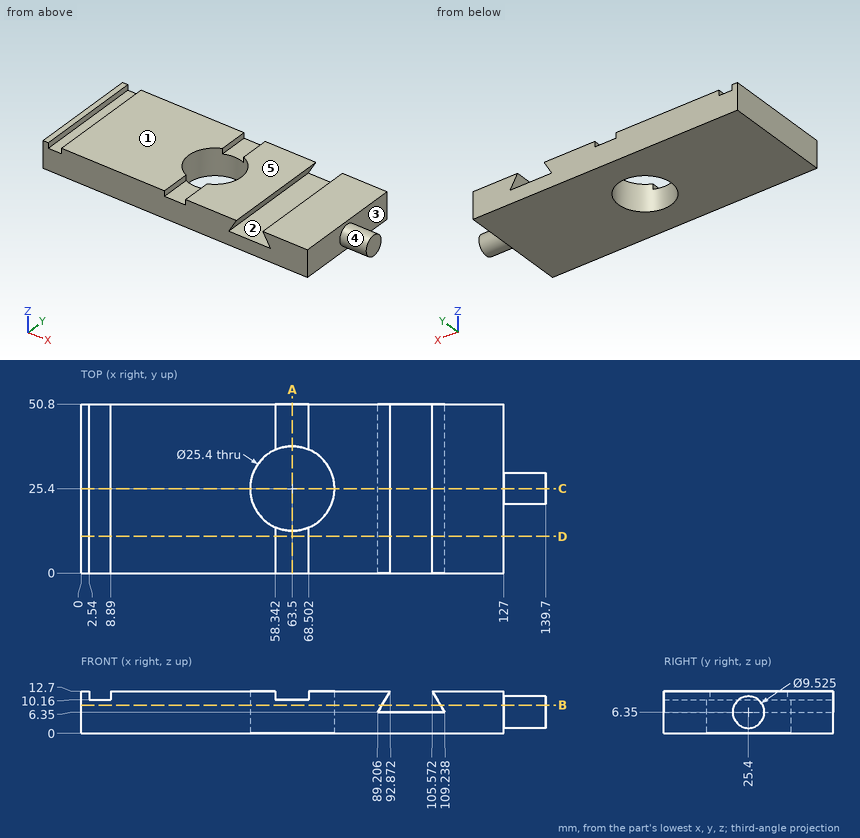
Part print with two shaded views. Sizes in mm from the minimum x, y, z corner. A direction names the side the tool comes from. Round coordinates to 2 decimals unless told otherwise and drop trailing zeros. Write each loop counter-clockwise with the first axis right and the second up, starting at its lowest first coordinate (ties: lowest second). Pieces come first, ordered by that corner, then holes. Notation, with made-up numbers: (77.5, 33) - (136.5, 33) arc R36 ccw to (136.5, 71) - close; hole circle Ø5 at (22, 18). An arc over 180 degrees is marked (long way). Answer as CSV lines item,"result".
Q1. Cut at B-B (z = 8.5). Write the cut outline in (x, y), and give its area (3 significant figures).
Report:
outline,"(0, 0) - (90.45, 0) - (90.45, 50.8) - (0, 50.8) - close; (108, 0) - (127, 0) - (127, 21.15) - (139.7, 21.15) - (139.7, 29.65) - (127, 29.65) - (127, 50.8) - (108, 50.8) - close; hole circle Ø25.4 at (63.5, 25.4)"
area,"5,160 mm^2"
Q2. Drop flat-ended pins along their axis: pin 1 (5 mm diameter, centred on x = 62.5, y = 5, fed in from +Z); pin 2 (3 mm diameter, centred on y = 30.5, z = 11.5, fed in from +X). Give the stop position or say it passes through.
Report:
pin 1,"stops at z = 10.16"
pin 2,"stops at x = 127"
Q3. Tool access for the marked faces 4 and 5: list every direction of +Z, -Z, +X, -X, +Y, -Y with a clear straight run to the whole face (end or side of a thin tool).
Report:
face 4,"+X"
face 5,"+Z, +X, -X, +Y, -Y"
Q4. Cut at A-A (x = 63.5). Write the cut outline in (y, z), and give its area (3 significant figures).
Report:
outline,"(0, 0) - (12.7, 0) - (12.7, 10.16) - (0, 10.16) - close; (38.1, 0) - (50.8, 0) - (50.8, 10.16) - (38.1, 10.16) - close"
area,"258 mm^2"
Q5. Drill centre lines: probe 1 along Y at (x, z) = (63.5, 6.5); probe 2 along X at (y, z) = (25.4, 3.5); probe 3 along X at (y, z) = (25.4, 7.25) (1 decimal). Where is each one in solid material? Low to high. Write a range as [from, to].
Report:
probe 1,"y = [0, 12.7], [38.1, 50.8]"
probe 2,"x = [0, 50.8], [76.2, 139.7]"
probe 3,"x = [0, 50.8], [76.2, 89.7], [108.7, 139.7]"
Q6. Cut at D-D (y = 11). Write the cut outline in (x, z), and give its area (3 significant figures).
Report:
outline,"(0, 0) - (127, 0) - (127, 12.7) - (105.57, 12.7) - (109.24, 6.35) - (89.21, 6.35) - (92.87, 12.7) - (68.5, 12.7) - (68.5, 10.16) - (58.34, 10.16) - (58.34, 12.7) - (8.89, 12.7) - (8.89, 10.16) - (2.54, 10.16) - (2.54, 12.7) - (0, 12.7) - close"
area,"1,470 mm^2"
Q7. Pull direction X, two halves, no side cores. Call the marked faces 1, 2 and 3: +X half, -X half, draft (parallel to the pull), parting line (faces both ways), or undercut.
Report:
face 1,"draft"
face 2,"undercut"
face 3,"+X half"
Q8. Cut at C-C (y = 25.4). Write the cut outline in (x, z), and give its area (3 significant figures).
Report:
outline,"(0, 0) - (50.8, 0) - (50.8, 12.7) - (8.89, 12.7) - (8.89, 10.16) - (2.54, 10.16) - (2.54, 12.7) - (0, 12.7) - close; (76.2, 0) - (127, 0) - (127, 1.59) - (139.7, 1.59) - (139.7, 11.11) - (127, 11.11) - (127, 12.7) - (105.57, 12.7) - (109.24, 6.35) - (89.21, 6.35) - (92.87, 12.7) - (76.2, 12.7) - close"
area,"1,290 mm^2"
